```python
from build123d import *

# Parameters (mm, degrees)
F1_DEPTH = 15
F2_D     = 13.2
F3_D     = 6.6
F4_R     = 10
F5_D     = 32
F6_D     = 5.5


with BuildPart() as f1:
    # F0 (on Front) → F1 (new body)
    with BuildSketch(Plane.XZ):
        Polygon((62.0740194619, 40.9148037434), (-57.9259805381, 40.9148037434), (-62.9259805381, 40.9148037434), (-62.9259805381, -29.0851962566), (-57.9259805381, -29.0851962566), (-7.9259805381, -29.0851962566), (-7.9259805381, -129.0851962566), (162.0740194619, -129.0851962566), (162.0740194619, -89.0851962566), (62.0740194619, -89.0851962566), align=None)
    extrude(amount=F1_DEPTH)

    # F2 (through all)
    with Locations(Plane(origin=(0, 0, 0), x_dir=(1, 0, 0), z_dir=(0, 1, 0))):
        with Locations((24.0740194619, 69.0851962566), (24.0740194619, 29.0851962566)):
            Hole(F2_D / 2)

    # F3 (through all)
    with Locations(Plane(origin=(0, 0, 0), x_dir=(1, 0, 0), z_dir=(0, 1, 0))):
        with Locations((24.0740194619, 109.0851962566), (74.0740194619, 109.0851962566), (124.0740194619, 109.0851962566)):
            Hole(F3_D / 2)

    # F4
    f4_edges = [f1.edges().sort_by_distance(p)[0] for p in [
        (62.074019, -7.5, 40.914804),
        (62.074019, -7.5, -89.085196),
        (162.074019, -7.5, -129.085196),
        (162.074019, -7.5, -89.085196),
        (-7.925981, -7.5, -129.085196),
        (-7.925981, -7.5, -29.085196),
        (-62.925981, -7.5, 40.914804),
        (-62.925981, -7.5, -29.085196),
    ]]
    fillet(f4_edges, radius=F4_R)

    # F5 (through all)
    with Locations(Plane(origin=(0, 0, 0), x_dir=(1, 0, 0), z_dir=(0, 1, 0))):
        with Locations((-29.9259805381, -0.9148037434)):
            Hole(F5_D / 2)

    # F6 (through all)
    with Locations(Plane(origin=(0, 0, 0), x_dir=(1, 0, 0), z_dir=(0, 1, 0))):
        with Locations((-53.4959805381, -24.4848037434), (-6.3559805381, -24.4848037434), (-6.3559805381, 22.6551962566), (-53.4959805381, 22.6551962566)):
            Hole(F6_D / 2)


solid = f1.part
```
Verification items for the finished model (mm, model axes). A direction names the side the tool comes from. Give positions to 0.01 mm unless a question says otherwise; leave off trailing zeros. Order: outer loops, then holes, each group sorted by start corner. A loop starts at its lowest first (then second) coordinate and runs counter-clockwise, first axis right, second up. Notation, with made-up numbers: (31, 87) -> (85, 87) arc R26 cw to (85, 126) -> close; hole circle Ø8 at (17.5, -19). An arc over 180 degrees is marked (long way). Use a Markdown table: item, result.
1) Mould release check, pull along X, two halves, no side actions. Record for faces 1 (the cylindrical face through (76.693, -7.605, -107.077)), 2 (the cylindrical face through (-60.07, -7.6, -26.08)), 3 (the cylindrical face through (159.07, -7.6, -91.94)): pulls with the +X half, pulls with the -X half, needs draft (parallel to the pull), parting line crosses it, or undercut.
Results:
| item | result |
|---|---|
| face 1 | undercut |
| face 2 | pulls with the -X half |
| face 3 | pulls with the +X half |
2) Section check B-B, the plane y = -9.25. Give the number of separate pieces and of enclosed holes in the cut face, then the cut area to 3 significant figures.
Results:
| item | result |
|---|---|
| separate pieces | 1 |
| enclosed holes | 10 |
| area | 18,400 mm² |
3) Section check A-A, the plane z = -65. Record the boundary of the cut face in (x, y).
Results:
| item | result |
|---|---|
| outline | (-7.93, -15) -> (18.89, -15) -> (18.89, 0) -> (-7.93, 0) -> close; (29.26, -15) -> (62.07, -15) -> (62.07, 0) -> (29.26, 0) -> close |
4) Section check D-D, the plane x = 88. Record the boundary of the cut face in (y, z), then the cut area to 3 significant figures.
Results:
| item | result |
|---|---|
| outline | (-15, -129.09) -> (0, -129.09) -> (0, -89.09) -> (-15, -89.09) -> close |
| area | 600 mm² |
5) Section check C-C, the plane z = 14. Record the boundary of the cut face in (x, y).
Results:
| item | result |
|---|---|
| outline | (-62.93, -15) -> (-39.13, -15) -> (-39.13, 0) -> (-62.93, 0) -> close; (-20.72, -15) -> (62.07, -15) -> (62.07, 0) -> (-20.72, 0) -> close |
6) Tool access check on faces 4 (the flat face through (62.074, -7, -25)), 5 (the cylindrical face through (-50.75, -7.61, -22.78)), 6 (the flat face through (-36, -7, -29.085)). Record the directions out of +Z, -Z, +X, -X, +Y, -Y that give a thin tool (end or side, any length) a straight path to the whole face; none if there is none.
Results:
| item | result |
|---|---|
| face 4 | +Z, +X, +Y, -Y |
| face 5 | +Y, -Y |
| face 6 | -Z, -X, +Y, -Y |
7) Material ranges on probe 1 along X at (y, z) = (-5.5, 22); probe 2 along Z at (x, y) = (26, -8.75); probe 3 along X at (y, z) = (-5, -24), recorded low to high.
Results:
| item | result |
|---|---|
| probe 1 | -62.93 to -54.67, -52.32 to -7.53, -5.18 to 62.07 |
| probe 2 | -129.09 to -111.76, -106.41 to -75.4, -62.77 to -35.4, -22.77 to 40.91 |
| probe 3 | -61.63 to -55.89, -51.1 to -8.75, -3.96 to 19.87, 28.28 to 62.07 |
8) Depth check by flat-ended pin: pin 1 Ø1.5 at (y, z) = (-9.5, -45) entering from +X; pin 2 Ø7.5 at (x, y) = (-28, -7.5) entering from -Z; pin 3 Ø5.5 at (x, z) = (124.07, -109.09) entering from +Y; pin 4 Ø4.5 at (x, y) = (103, -9) entering from +Z. Enter the tip coordinate at first touch or a pass-through.
Results:
| item | result |
|---|---|
| pin 1 | x = 62.07 |
| pin 2 | z = -29.09 |
| pin 3 | through |
| pin 4 | z = -89.09 |
